Geometry: final body of the model. Coordinates: model frame, mm. A direction names the side the tool comes from. Round coordinates to 2 decimals unless told otherwise and drop trailing zeros. Loops run counter-clockwise (first coordinate to the right, second up) from the corner with the lowest first, then second, coordinate; pieces in that order, holes last. Notation, with made-up numbers: (-12, 23) - (33, 23) arc R19 cw to (33, 38) - close; hole circle Ø5 at (8, 63.5). An arc over 180 degrees is marked (long way). Write item = value, one per line. Start each with the question number.
Item 1: Section B-B (x = 21.15). Return loops of the section in (y, z).
Item 2: Section C-C (y = 29.5). Return loops of the section in (x, z), plus the area to 3 significant figures.
Item 3: Section D-D (z = -35). Return loops of the section in (x, y), plus the area to 3 significant figures.
Item 4: Line query: line 1 (X direction, y = 5, z = 8); line 2 (Z direction, x = 19, y = 28.5). Output: solid intervals per line, ascending. Write a range as from..to.
Item 5: Section A-A (z = -18). Return loops of the section in (x, y).
Item 6: First-contact query: pin 1 (0.9 mm diameter, centred on x = 37.5, y = 37.5, fed in from -Z); pin 2 (3.5 mm diameter, centred on x = 6, y = 37.5, fed in from +Z); pin 3 (1.5 mm diameter, centred on x = 5, y = 36.5, fed in from -Z); pin 4 (12 mm diameter, centred on x = 10.5, y = 24.5, fed in from +Z). Flat tips, straight axial feed; report the tip coordinate or a pass-through.
Item 7: Access query for faces 5 (the cylindrical face through (38.15, 5.72, -38.03)), 6 (the flat face through (2.79, 2.86, -36.2)), 7 (the cylindrical face through (5.325, 35.186, 7.781)), 8 (the flat face through (39.51, 39.44, -36.2)), 9 (the flat face through (3, 39, 0)). Directions: +Z, -Z, +X, -X, +Y, -Y. A direction counts if a zero-diameter tool reaches every point of the face in a straight line with its end or side. Return the directions, or none.
Item 8: Draft query along Z for faces 1 (the flat face through (39, 39, -32.5)), 2 (the flat face through (0, 21, -15)), 3 (the flat face through (37, 6, -36)), 4 (the flat face through (3, 3, -32.5)). Return one class per face: pulls with the +Z half, pulls with the -Z half, needs draft (parallel to the pull), parting line crosses it, or undercut.
Autodesk Inventor part; units mm, degrees
ref_plane "YZ Plane" through (0, 0, 0) normal (1, 0, 0) x (0, 1, 0)
ref_plane "XZ Plane" through (0, 0, 0) normal (0, 1, 0) x (-1, 0, 0)
ref_plane "XY Plane" through (0, 0, 0) normal (0, 0, 1) x (1, 0, 0)
sketch "Эскиз1" plane through (0, 0, 0) normal (0, 0, 1) x (1, 0, 0)
  line L0 (0, 0) -> (42.3, 0)
  line L1 (42.3, 0) -> (42.3, 42.3)
  line L2 (42.3, 42.3) -> (0, 42.3)
  line L3 (0, 42.3) -> (0, 0)
  dimension "d0" = 42.3
  dimension "d1" = 42.3
extrude "Выдавливание1" add sketch "Эскиз1" along normal blind 10
sketch "Эскиз2" plane through (0, 0, 10) normal (0, 0, 1) x (1, 0, 0)
  circle A0 centre (5.65, 5.65) radius 1.5
  circle A1 centre (5.65, 36.65) radius 1.5
  line L0 (0, 0) -> (42.3, 0)
  line L1 (42.3, 0) -> (42.3, 42.3)
  line L2 (36.65, 5.65) -> (36.65, 36.65)
  circle A2 centre (36.65, 36.65) radius 1.5
  circle A3 centre (36.65, 5.65) radius 1.5
  point P0 (0, 42.3)
  dimension "d6" = 3
  dimension "d7" = 3
  dimension "d12" = 31
  dimension "d13" = 3
  dimension "d14" = 3
extrude "Выдавливание2" cut sketch "Эскиз2" against normal blind 4.5
thread "Резьба1"
thread "Резьба2"
thread "Резьба3"
thread "Резьба4"
sketch "Эскиз3" plane through (0, 0, 10) normal (0, 0, 1) x (1, 0, 0)
  line L0 (0, 42.3) -> (0, 0)
  line L1 (0, 42.3) -> (0, 37.8)
  line L2 (0, 0) -> (42.3, 0)
  line L3 (0, 0) -> (0, 4.5)
  line L4 (0, 0) -> (4.5, 0)
  line L5 (4.5, 0) -> (0, 4.5)
  line L6 (42.3, 42.3) -> (0, 42.3)
  line L7 (0, 42.3) -> (4.5, 42.3)
  line L8 (4.5, 42.3) -> (0, 37.8)
  line L9 (42.3, 42.3) -> (37.8, 42.3)
  line L10 (42.3, 0) -> (42.3, 42.3)
  line L11 (42.3, 42.3) -> (42.3, 37.8)
  line L12 (42.3, 37.8) -> (37.8, 42.3)
  line L13 (42.3, 0) -> (37.8, 0)
  line L14 (42.3, 0) -> (42.3, 4.5)
  line L15 (42.3, 4.5) -> (37.8, 0)
  dimension "d27" = 4.5
  dimension "d28" = 4.5
  dimension "d29" = 4.5
  dimension "d30" = 4.5
  dimension "d31" = 4.5
  dimension "d32" = 4.5
extrude "Выдавливание3" cut sketch "Эскиз3" against normal blind 10 contours L6 L8 L0 | L5 L2 L0 | L6 L10 L12 | L15 L10 L2
chamfer "Фаска1" distance 0.5 angle 45 1 edges at (4.5, 42.3, 5)
chamfer "Фаска2" distance 0.5 angle 45 7 edges at (0, 37.8, 5) (37.8, 42.3, 5) (42.3, 37.8, 5) (42.3, 4.5, 5) (37.8, 0, 5) (4.5, 0, 5) (0, 4.5, 5)
sketch "Эскиз5" plane through (0, 0, 0) normal (0, 0, -1) x (-1, 0, 0)
  line L0 (0, 0) -> (-42.3, 0)
  line L1 (-42.3, 0) -> (-42.3, 42.3)
  line L2 (-42.3, 42.3) -> (0, 42.3)
  line L3 (0, 42.3) -> (0, 0)
  line L4 (-42.3, 42.3) -> (-42.3, 35.3)
  line L5 (-42.3, 5) -> (-42.3, 37.3)
  line L6 (-42.3, 42.3) -> (-35.3, 42.3)
  line L7 (-37.3, 42.3) -> (-5, 42.3)
  line L8 (-35.3, 42.3) -> (-42.3, 35.3)
  line L9 (-42.3, 0) -> (-35.3, 0)
  line L10 (-42.3, 0) -> (-42.3, 7)
  line L11 (-42.3, 7) -> (-35.3, 0)
  line L12 (0, 0) -> (-7, 0)
  line L13 (-5, 0) -> (-37.3, 0)
  line L14 (0, 0) -> (0, 7)
  line L15 (0, 7) -> (-7, 0)
  line L16 (0, 42.3) -> (-7, 42.3)
  line L17 (-7, 42.3) -> (0, 35.3)
  line L18 (0, 37.3) -> (0, 5)
  dimension "d41" = 42.3
  dimension "d42" = 42.3
  dimension "d43" = 7
  dimension "d44" = 7
  dimension "d45" = 7
  dimension "d46" = 7
  dimension "d47" = 7
  dimension "d48" = 7
  dimension "d49" = 7
extrude "Выдавливание4" add sketch "Эскиз5" along normal blind 32.5 contours L0 L11 L1 L8 L2 L17 L3 L15
chamfer "Фаска3" distance 0.5 angle 45 8 edges at (0, 35.3, -16.25) (7, 42.3, -16.25) (0, 7, -16.25) (7, 0, -16.25) (42.3, 35.3, -16.25) (35.3, 42.3, -16.25) (42.3, 7, -16.25) (35.3, 0, -16.25)
sketch "Эскиз10" plane through (0, 0, -32.5) normal (0, 0, -1) x (-1, 0, 0)
  line L0 (0, 0) -> (-42.3, 0)
  line L1 (-42.3, 0) -> (-42.3, 42.3)
  line L2 (-42.3, 42.3) -> (0, 42.3)
  line L3 (0, 42.3) -> (0, 0)
  line L4 (-42.3, 42.3) -> (-36.65, 42.3)
  line L5 (-42.3, 42.3) -> (-42.3, 36.65)
  line L6 (-42.3, 36.65) -> (-36.65, 42.3)
  line L7 (0, 42.3) -> (-5.65, 42.3)
  line L8 (0, 42.3) -> (0, 36.65)
  line L9 (0, 36.65) -> (-5.65, 42.3)
  line L10 (-37.3, 42.3) -> (-5, 42.3)
  line L11 (0, 0) -> (-5.65, 0)
  line L12 (0, 0) -> (0, 5.65)
  line L13 (0, 7.5) -> (0, 5)
  line L14 (0, 5.65) -> (-5.65, 0)
  line L15 (-42.3, 0) -> (-42.3, 5.65)
  line L16 (-42.3, 0) -> (-36.65, 0)
  line L17 (-35.6536, 0.3536) -> (-41.9464, 6.6464)
  line L18 (-36.65, 0) -> (-42.3, 5.65)
  dimension "d57" = 42.3
  dimension "d58" = 42.3
  dimension "d59" = 5.65
  dimension "d60" = 5.65
  dimension "d61" = 5.65
  dimension "d62" = 5.65
  dimension "d63" = 5.65
  dimension "d64" = 5.65
  dimension "d65" = 5.65
  dimension "d66" = 5.65
extrude "Выдавливание5" add sketch "Эскиз10" along normal blind 7.5 contours L0 L18 L1 L6 L2 L9 L3 L14
chamfer "Фаска4" distance 0.5 angle 45 8 edges at (0, 36.65, -36.25) (5.65, 42.3, -36.25) (0, 5.65, -36.25) (5.65, 0, -36.25) (36.65, 0, -36.25) (42.3, 5.65, -36.25) (36.65, 42.3, -36.25) (42.3, 36.65, -36.25)
sketch "Эскиз11" plane through (0, 0, -40) normal (0, 0, -1) x (-1, 0, 0)
  circle A0 centre (-5.65, 5.65) radius 1.5
  circle A1 centre (-5.65, 5.65) radius 1.5
  circle A2 centre (-36.65, 5.65) radius 1.5
  circle A3 centre (-36.65, 5.65) radius 1.5
  circle A4 centre (-36.65, 36.65) radius 1.5
  circle A5 centre (-36.65, 36.65) radius 1.5
  circle A6 centre (-5.65, 36.65) radius 1.5
  circle A7 centre (-5.65, 36.65) radius 1.5
  point P0 (0, 0)
extrude "Выдавливание6" cut sketch "Эскиз11" against normal blind 4
thread "Резьба5"
thread "Резьба6"
thread "Резьба7"
thread "Резьба8"
sketch "Эскиз12" plane through (0, 0, 10) normal (0, 0, 1) x (1, 0, 0)
  line L0 (0, 0) -> (42.3, 0)
  line L1 (42.3, 0) -> (42.3, 42.3)
  line L2 (42.3, 42.3) -> (0, 42.3)
  line L3 (0, 42.3) -> (0, 0)
  line L4 (0, 42.3) -> (42.3, 0)
  line L5 (0, 0) -> (42.3, 42.3)
  circle A0 centre (21.15, 21.15) radius 11
  dimension "d82" = 42.3
  dimension "d83" = 42.3
  dimension "d84" = 22
extrude "Выдавливание7" add sketch "Эскиз12" along normal blind 2 contours A0 L4 L5 | L5 L4 A0 | L4 L5 A0 | A0 L5 L4
sketch "Эскиз13" plane through (21.15, 21.15, 12) normal (0, 0, 1) x (1, 0, 0)
  circle A0 centre (0, 0) radius 2.5
  point P0 (-21.15, -21.15)
  dimension "d87" = 5
extrude "Выдавливание8" add sketch "Эскиз13" along normal blind 22
properties part number "Nema17"
Taken from the geometry:
q1.outline = (0, -40) - (42.3, -40) - (42.3, 10) - (32.15, 10) - (32.15, 12) - (23.65, 12) - (23.65, 34) - (18.65, 34) - (18.65, 12) - (10.15, 12) - (10.15, 10) - (0, 10) - close
q2.outline = (0, -40) - (42.3, -40) - (42.3, 10) - (28.31, 10) - (28.31, 12) - (13.99, 12) - (13.99, 10) - (0, 10) - close
q2.area = 2,140 mm^2
q3.outline = (0, 6.15) - (0.35, 5.3) - (5.3, 0.35) - (6.15, 0) - (36.15, 0) - (37, 0.35) - (41.95, 5.3) - (42.3, 6.15) - (42.3, 36.15) - (41.95, 37) - (37, 41.95) - (36.15, 42.3) - (6.15, 42.3) - (5.3, 41.95) - (0.35, 37) - (0, 36.15) - close
q3.area = 1,720 mm^2
q4.line_1 = 0..4.3, 7..35.3, 38..42.3
q4.line_2 = -40..12
q5.outline = (0, 7.5) - (0.35, 6.65) - (6.65, 0.35) - (7.5, 0) - (34.8, 0) - (35.65, 0.35) - (41.95, 6.65) - (42.3, 7.5) - (42.3, 34.8) - (41.95, 35.65) - (35.65, 41.95) - (34.8, 42.3) - (7.5, 42.3) - (6.65, 41.95) - (0.35, 35.65) - (0, 34.8) - close
q6.pin_1 = -40
q6.pin_2 = 10
q6.pin_3 = -36
q6.pin_4 = 12
q7.face_5 = -Z
q7.face_6 = -Z, -X, -Y
q7.face_7 = +Z
q7.face_8 = -Z, +X, +Y
q7.face_9 = -X, +Y
q8.face_1 = undercut
q8.face_2 = needs draft
q8.face_3 = pulls with the -Z half
q8.face_4 = undercut
